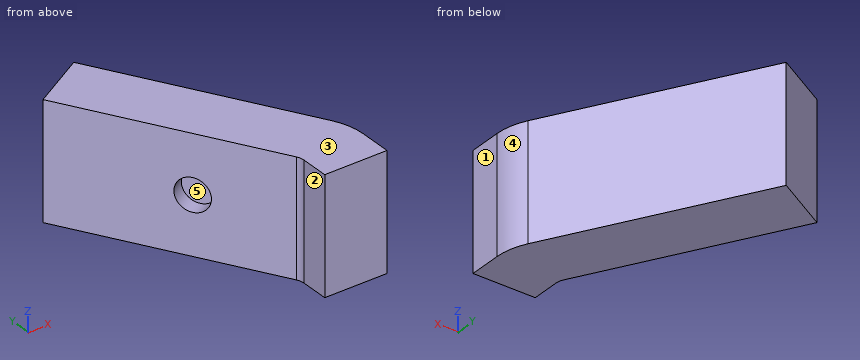
```python
from build123d import *

# Parameters (mm, degrees)
F0_W      = 105.1309853792
F0_H      = 195.6836879253
F1_DEPTH  = 53.975
F1_FACE_W = 105.1309853792
F1_FACE_H = 195.6836879253
F2_ANGLE  = 30
F3_DEPTH  = 381
F4_R      = 25.4
F5_R      = 27.7266508926
F6_DEPTH  = 25.4


with BuildPart() as f1:
    # F0 (on Front) → F1 (new body)
    with BuildSketch(Plane.XZ):
        with Locations((-20.0917944312, 0)):
            Rectangle(F0_W, F0_H)
    extrude(amount=F1_DEPTH)

    # F1_face (on face) → F2 (revolve)
    with BuildSketch(Plane(origin=(-20.0917944312, 0, 0), x_dir=(1, 0, 0), z_dir=(0, 1, 0))):
        Rectangle(F1_FACE_W, F1_FACE_H)
    revolve(axis=Axis((-72.6572871208, 0, 0), (0, 0, 1)), revolution_arc=F2_ANGLE)

    # F3 (add): a face of the model
    f3_faces = [f1.faces().sort_by_distance(p)[0] for p in [
        (-27.1342350892, 26.2827463448, 0),
    ]]
    extrude(f3_faces, amount=F3_DEPTH)

    # F4
    f4_edges = [f1.edges().sort_by_distance(p)[0] for p in [
        (-72.657287, 0, 0),
    ]]
    fillet(f4_edges, radius=F4_R)

    # F5 (on face) → F6 (cut)
    with BuildSketch(Plane(origin=(-54.4929653406, -31.4615282083, 0), x_dir=(0.5, -0.8660254038, 0), z_dir=(-0.8660254038, -0.5, 0))):
        with Locations((-196.3157951832, 0)):
            Circle(F5_R)
    extrude(amount=-F6_DEPTH, mode=Mode.SUBTRACT)


solid = f1.part
```
Here's how the part is built. I have some questions about the finished solid (model axes, mm). Face numbers are marked on the shaded views. A direction names the side the tool comes from. Coordinates: 2 decimals unless noted, no trailing zeros. Write each loop counter-clockwise with the first axis right and the second up, starting at its lowest first coordinate (ties: lowest second). Pieces come first, ordered by that corner, then holes. Notation, with made-up numbers: (-25, 4.5) -> (11, 4.5) arc R35 ccw to (11, 37.5) -> close; hole circle Ø2 at (27.5, -29). An arc over 180 degrees is marked (long way). Use a Markdown table: item, result. Add a question column.
(1) If we section it at C-C, the plane z = -10: Write out the boundary of the cut face in (x, y) (1 decimal).
(2) For the marked faces 1 and 2, which set-ups out of +Z, -Z, +X, -X, +Y, -Y let a thin tool reach every point of the face, with its end or its side?
(3) If we section it at A-A, the plane z = -79: Write out the boundary of the cut face in (x, y) (1 decimal).
(4) We'd pull the mould along Z, two halves only. Please class the marked faces 3, 4 and 5: +Z half, -Z half, draft (parallel to the pull), parting line (faces both ways), or undercut.
(5) Please list where these lines run through material, in increasing order: line 1 (X direction, y = -4.5, z = 19.5); line 2 (Y direction, x = -128.5, z = -8.5); line 3 (X direction, y = 170.5, z = 8.5).
(6) If we section it at B-B, the plane x = -21: Write out the boundary of the cut face in (y, z) (3 decimals), and give its area (3 significant figures).
(7) I'm going to push flat-ended pins straight in: P1, Ø14, axis at y = -23, z = 46.5, coming from the -X side; P2, Ø10, axis at y = 135.5, z = -66, coming from the +X side; P3, Ø6, axis at y = 290, z = -25, coming from the +X side. Where does each tip first touch, or does it pass through?
(8) If we section it at D-D, the plane y = 342.5: Write out the boundary of the cut face in (x, z), and give its area (3 significant figures).
Outcome:
| question | item | result |
|---|---|---|
| 1 | outline | (-263.2, 330) -> (-165.6, 160.9) -> (-143.6, 173.6) -> (-117.7, 128.9) -> (-139.7, 116.2) -> (-76.1, 5.9) arc R25.4 cw to (-72.7, -6.8) -> (-72.7, -54) -> (32.5, -54) -> (32.5, 0) arc R105.1 ccw to (18.4, 52.6) -> (-172.1, 382.5) -> close |
| 2 | face 1 | +Z, -Z, +X, +Y, -Y |
| 2 | face 2 | +Z, -Z, -X, -Y |
| 3 | outline | (-263.2, 330) -> (-76.1, 5.9) arc R25.4 cw to (-72.7, -6.8) -> (-72.7, -54) -> (32.5, -54) -> (32.5, 0) arc R105.1 ccw to (18.4, 52.6) -> (-172.1, 382.5) -> close |
| 4 | face 3 | +Z half |
| 4 | face 4 | draft |
| 4 | face 5 | undercut |
| 5 | line 1 | x = -72.76 to 32.47 |
| 5 | line 2 | y = 96.72 to 122.02, 147.52 to 306.98 |
| 5 | line 3 | x = -171.1 to -150.1, -141.77 to -49.7 |
| 6 | outline | (-53.975, -97.842) -> (120.789, -97.842) -> (120.789, 97.842) -> (-53.975, 97.842) -> close |
| 6 | area | 34,200 mm^2 |
| 7 | P1 | stops at x = -72.66 |
| 7 | P2 | stops at x = -26.61 |
| 7 | P3 | stops at x = -116.96 |
| 8 | outline | (-241.43, -97.84) -> (-149, -97.84) -> (-149, 97.84) -> (-241.43, 97.84) -> close |
| 8 | area | 18,100 mm^2 |
